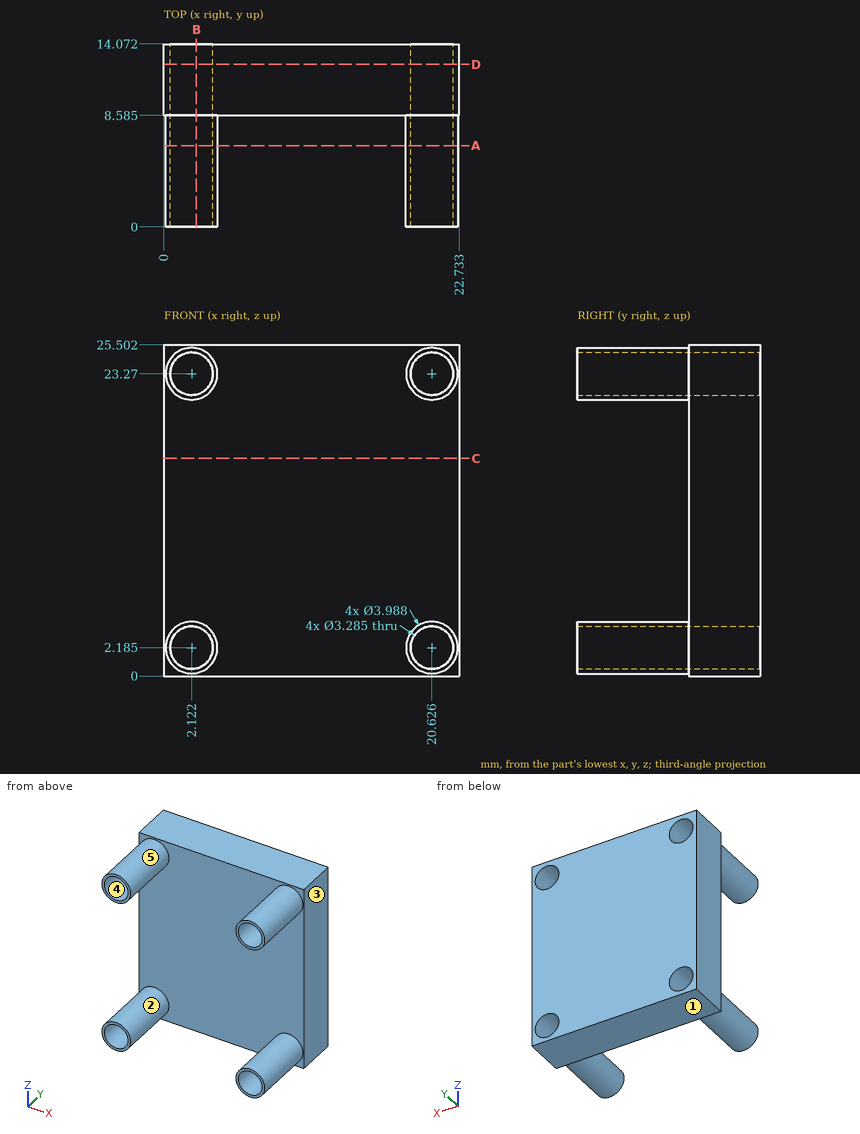
The drawing under review shows one solid part. Ordinate dimensions are in mm from its lowest x, y, z. A direction names the side the tool comes from. Round coordinates to 2 decimals unless told otherwise and drop trailing zeros. Loops run counter-clockwise (first coordinate to the right, second up) from the corner with the lowest first, then second, coordinate; pieces in that order, holes last. Notation, with made-up numbers: M -36,59 L -29,59 A23 ccw -29,81 Z; hole C 4,58 d8. An arc over 180 degrees is marked long. Answer as CSV lines item,"result". Start each with the question number.
Item 1: Insertion check: P1, Ø3, axis at x = 3.5, z = 13, coming from the -Y side (1 decimal). The pin has a flat end and moves straight along its axis. Give the tip position at first contact, or say it passes through.
Item 2: For the marked faces 4 and 5, list the 3-axis set-ups (+Z, -Z, +X, -X, +Y, -Y) from which the entire face can be reached by the end or side of a thin tool; tool diameter is ignored.
Item 3: Consider section D-D (y = 12.5). Write out the cut boundary in (x, z) (1 decimal).
Item 4: Consider section C-C (z = 16.75). Write out the cut boundary in (x, y) (1 decimal).
Item 5: Consider section A-A (y = 6.25). Write out the cut boundary in (x, z) (1 decimal).
Item 6: Mouldability with a two-part tool opening along Z and no side actions: class the marked faces 1, 2 and 3 as released by +Z, released by -Z, zero draft, split by the parting line, or undercut.
Item 7: Consider section B-B (x = 2.5). State how many separate pieces and enclosed holes the cut face has, then the cut area to 3 significant figures.
Item 8: Wall thickness on line 1 (Z direction, x = 2, y = 8.75); line 2 (X direction, y = 2.75, z = 23.5) (1 decimal); line 3 (Y direction, x = 6, z = 6.5) (1 decimal): over which ranges is each line inside the solid? List them lowest first. Write a range as [from, to].
Answer:
1,P1,"stops at y = 8.6"
2,face 4,"+Y, -Y"
2,face 5,"-Y"
3,outline,"M 0,0 L 22.7,0 L 22.7,25.5 L 0,25.5 Z; hole C 2.1,2.2 d3.3; hole C 2.1,23.3 d3.3; hole C 20.6,2.2 d3.3; hole C 20.6,23.3 d3.3"
4,outline,"M 0,8.6 L 22.7,8.6 L 22.7,14.1 L 0,14.1 Z"
5,outline,"C 2.1,2.2 d4; C 2.1,23.3 d4; C 20.6,2.2 d4; C 20.6,23.3 d4; hole C 2.1,2.2 d3.3; hole C 2.1,23.3 d3.3; hole C 20.6,2.2 d3.3; hole C 20.6,23.3 d3.3"
6,face 1,"released by -Z"
6,face 2,"undercut"
6,face 3,"zero draft"
7,separate pieces,"3"
7,enclosed holes,"0"
7,area,"117 mm^2"
8,line 1,"z = [0, 0.55], [3.82, 21.63], [24.91, 25.5]"
8,line 2,"x = [0.1, 0.5], [3.7, 4.1], [18.6, 19], [22.3, 22.6]"
8,line 3,"y = [8.6, 14.1]"
